Input: part model. Units: mm. Frame: model coordinates. A direction names the side the tool comes from. Give positions to 0.01 mm unless a question says otherwise; leave off trailing zeros. Loops run counter-clockwise (first coordinate to the right, second up) from the corner with the lowest first, then second, coordinate; pieces in that order, holes last. Notation, with made-up numbers: (85, 19.5) -> (115, 19.5) arc R11 cw to (115, 33.5) -> close; hole circle Ø10 at (34, 79). An arc over 180 degrees is marked (long way). Answer as a JSON object with one key per item and string values.
```python
from build123d import *

# Parameters (mm, degrees)
SALIENTE_EXTRUIR1_DEPTH = 3
CROQUIS3_R              = 5
CORTAR_EXTRUIR2_DEPTH   = 10
REDONDEO1_R             = 10
CROQUIS2_R              = 2.75
SALIENTE_EXTRUIR2_DEPTH = 9


with BuildPart() as part:
    # Croquis1 → Saliente-Extruir1 (new body)
    with BuildSketch(Plane.XY):
        with BuildLine():
            Line((-13.118348224, -13.346885602), (-5.358962429, -8.729934305))
            ThreePointArc((-5.358962429, -8.729934305), (0, -10.243545836), (5.358962429, -8.729934305))
            Line((5.358962429, -8.729934305), (13.118348224, -13.346885602))
            ThreePointArc((13.118348224, -13.346885602), (19.97194541, -11.606711584), (18.231771393, -4.753114398))
            Line((18.231771393, -4.753114398), (10.243545836, 0))
            ThreePointArc((10.243545836, 0), (8.83594818, 5.182301714), (5, 8.94037087))
            Line((5, 8.94037087), (5, 18.2))
            ThreePointArc((5, 18.2), (0, 23.2), (-5, 18.2))
            Line((-5, 18.2), (-5, 8.94037087))
            ThreePointArc((-5, 8.94037087), (-8.83594818, 5.182301714), (-10.243545836, 0))
            Line((-10.243545836, 0), (-18.231771393, -4.753114398))
            ThreePointArc((-18.231771393, -4.753114398), (-19.97194541, -11.606711584), (-13.118348224, -13.346885602))
        make_face()
    extrude(amount=SALIENTE_EXTRUIR1_DEPTH)

    # Croquis3 → Cortar-Extruir2 (cut)
    with BuildSketch(Plane.XY.offset(3)):
        Circle(CROQUIS3_R)
    extrude(amount=-CORTAR_EXTRUIR2_DEPTH, mode=Mode.SUBTRACT)

    # Redondeo1
    redondeo1_edges = [part.edges().sort_by_distance(p)[0] for p in [
        (-10.243545836, 0, 1.5),
        (-5, 8.94037087, 1.5),
        (5, 8.94037087, 1.5),
        (10.243545836, 0, 1.5),
        (5.358962429, -8.729934305, 1.5),
        (-5.358962429, -8.729934305, 1.5),
    ]]
    fillet(redondeo1_edges, radius=REDONDEO1_R)

    # Croquis2 → Saliente-Extruir2 (add)
    with BuildSketch(Plane.XY.offset(3)):
        with Locations((0, 18.2)):
            Circle(CROQUIS2_R)
        with Locations((15.675059808, -9.05)):
            Circle(CROQUIS2_R)
        with Locations((-15.675059808, -9.05)):
            Circle(CROQUIS2_R)
    extrude(amount=SALIENTE_EXTRUIR2_DEPTH)


solid = part.part
```
Q1. Ray query, line 1 along Y through (x, z) = (0, 1.2); line 2 along Y through (x, z) = (15.5, 9.5); line 3 along Z through (x, y) = (4, 21). Return the intervals inside material, ascending.
Evaluation:
{"line 1": "y = -10.24 to -5, 5 to 23.2", "line 2": "y = -11.79 to -6.31", "line 3": "z = 0 to 3"}
Q2. Section D-D, the plane y = 0. Return the cut outline in (x, z).
Evaluation:
{"outline": "(-11.46, 0) -> (-5, 0) -> (-5, 3) -> (-11.46, 3) -> close; (5, 0) -> (11.46, 0) -> (11.46, 3) -> (5, 3) -> close"}
Q3. Section C-C, the plane y = -9.05. Return the cut outline in (x, z), then the cut area to 3 significant figures.
Evaluation:
{"outline": "(-20.68, 0) -> (20.68, 0) -> (20.68, 3) -> (18.43, 3) -> (18.43, 12) -> (12.93, 12) -> (12.93, 3) -> (-12.93, 3) -> (-12.93, 12) -> (-18.43, 12) -> (-18.43, 3) -> (-20.68, 3) -> close", "area": "223 mm2"}
Q4. Draft query along X for faces 4 (the flat face through (11.268, -12.246, 1.479)), 5 (the cylindrical face through (11.47, -0.01, 1.52)), 6 (the flat face through (-16, -9, 12)), 7 (the flat face through (-16.153, -3.516, 1.479)). Return one class per face: +X half, -X half, draft (parallel to the pull), parting line (faces both ways), or undercut.
Evaluation:
{"face 4": "undercut", "face 5": "+X half", "face 6": "draft", "face 7": "-X half"}
Q5. Section A-A, the plane x = 0. Return the cut outline in (y, z).
Evaluation:
{"outline": "(-10.24, 0) -> (-5, 0) -> (-5, 3) -> (-10.24, 3) -> close; (5, 0) -> (23.2, 0) -> (23.2, 3) -> (20.95, 3) -> (20.95, 12) -> (15.45, 12) -> (15.45, 3) -> (5, 3) -> close"}
Q6. Access query for faces 1 (the flat face through (-11.319, -12.276, 1.479)), 2 (the cylindrical face through (-13.052, -8.224, 7.437)), 3 (the flat face through (-5, 16, 1)). Directions: +Z, -Z, +X, -X, +Y, -Y. A direction counts if a zero-diameter tool reaches every point of the face in a straight line with its end or side. Return the directions, or none.
Evaluation:
{"face 1": "+Z, -Z, -Y", "face 2": "+Z", "face 3": "+Z, -Z, -X, +Y"}
Q7. Section B-B, the plane z = 1.75. Return the cut outline in (x, y), then the cut area to 3 significant figures.
Evaluation:
{"outline": "(-18.23, -4.75) arc R5 ccw to (-13.12, -13.35) -> (-9.47, -11.18) arc R10 cw to (-2.2, -10) arc R10.24 ccw to (2.2, -10) arc R10 cw to (9.47, -11.18) -> (13.12, -13.35) arc R5 ccw to (18.23, -4.75) -> (14.13, -2.31) arc R10 cw to (9.74, 3.18) arc R10.24 ccw to (7.59, 6.88) arc R10 cw to (5, 13.59) -> (5, 18.2) arc R5 ccw to (-5, 18.2) -> (-5, 13.59) arc R10 cw to (-7.59, 6.88) arc R10.24 ccw to (-9.74, 3.18) arc R10 cw to (-14.13, -2.31) -> close; hole circle Ø10 at (0, 0)", "area": "633 mm2"}
Q8. Pin query (flat end, axial travel): pin 1 (5 mm diameter, centred on x = -12, y = 0, fed in from -Z); pin 2 (2 mm diameter, centred on x = -16, z = 5.5, fed in from +Y); pin 3 (0.9 mm diameter, centred on y = 15, z = 1, fed in from -X); pin 4 (1.5 mm diameter, centred on y = -8, z = 3.5, fed in from +X). Return the tip coordinate at first contact, or that it passes through.
Evaluation:
{"pin 1": "stops at z = 0", "pin 2": "stops at y = -6.3", "pin 3": "stops at x = -5", "pin 4": "stops at x = 20.65"}
